Geometry check sheet. Reference: the model listing, model coordinates, mm. Face numbers are marked on the shaded views. A direction names the side the tool comes from. Round coordinates to 2 decimals unless told otherwise and drop trailing zeros. Write each loop counter-clockwise with the first axis right and the second up, starting at its lowest first coordinate (ties: lowest second). Pieces come first, ordered by that corner, then holes. Notation, with made-up numbers: M 3.5,-12.5 L 57.5,-12.5 A29 ccw 57.5,11.5 Z; hole C 40.25,-9.75 d5. An arc over 180 degrees is marked long. Put each result on its own line as item: value. Start each with the question number.
(1) Tool access check on the marked faces 1 and 2. Record the directions out of +Z, -Z, +X, -X, +Y, -Y that give a thin tool (end or side, any length) a straight path to the whole face; none if there is none.
(2) Material ranges on probe 1 along Y at (x, z) = (-11, -5); probe 2 along Y at (x, z) = (-11, -2.4); probe 3 along X at (y, z) = (10, -6.5), recorded low to high.
(3) Gauge pin test, flat ends, axial feed: pin 1 (12 mm diameter, centred on y = 13.5, z = -27, fed in from -X); pin 2 (1.5 mm diameter, centred on x = -31.5, y = 13, fed in from +Z); pin 3 (6.5 mm diameter, centred on y = 13, z = -5.5, fed in from -X). Record the tip position at first contact, or that the pin passes through.
(4) Section check A-A on y = 10. Record the cut outline in (x, z).
(5) Section check B-B on x = -11. Record the cut outline in (y, z).
(6) Section check C-C on y = 3.5. Record the cut outline in (x, z).
(7) Section check D-D on z = -9. Record the cut outline in (x, y), then the cut area to 3 significant figures.
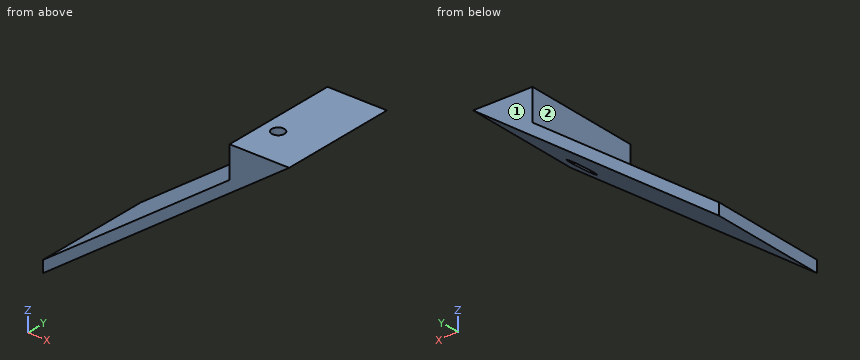
from build123d import *

# Parameters (mm, degrees)
EXTRUDE_1_DEPTH     = 30
SKETCH_2_R          = 1.6
CUT_EXTRUDE_1_DEPTH = 83.29890272
CUT_EXTRUDE_2_REACH = 82.696
SKETCH_3_R          = 3


with BuildPart() as part:
    # 草图1 → 凸台-拉伸1 (new body)
    with BuildSketch(Plane(origin=(0, 0, 0), x_dir=(1, 0, 0), z_dir=(0, 1, 0))):
        Polygon((0, 0), (-62, 45.045636736), (-62, 42.07907359), (-15, 7.931574774), (-15, 0), align=None)
    extrude(amount=EXTRUDE_1_DEPTH)

    # 草图2 → 切除-拉伸1 (cut, through all)
    with BuildSketch(Plane.XY):
        with Locations((-11, 10)):
            Circle(SKETCH_2_R)
    extrude(amount=-CUT_EXTRUDE_1_DEPTH, mode=Mode.SUBTRACT)

    # 切除-拉伸2: up to this plane
    cut_extrude_2_end = Plane(origin=(0, 30, 0), z_dir=(-0.5877852522924716, 0, 0.8090169943749486))
    # 草图3 → 切除-拉伸2 (cut, up to the surface)
    with BuildSketch(Plane.XY.offset(-3), mode=Mode.PRIVATE) as cut_extrude_2_sk1:
        with Locations((-11, 10)):
            Circle(SKETCH_3_R)
    cut_extrude_2_tool1 = split(extrude(cut_extrude_2_sk1.sketch, amount=-CUT_EXTRUDE_2_REACH, mode=Mode.PRIVATE), bisect_by=cut_extrude_2_end, keep=Keep.BOTH, mode=Mode.PRIVATE)
    add(cut_extrude_2_tool1.solids().sort_by_distance((-11, 10, -3))[0], mode=Mode.SUBTRACT)


solid = part.part
Answers follow:
1. face 1: +Z, -Z, +X, -X, +Y
1. face 2: +Z, -X, +Y, -Y
2. probe 1: y = 0 to 7, 13 to 30
2. probe 2: y = 0 to 8.4, 11.6 to 30
2. probe 3: x = -15 to -14
3. pin 1: stops at x = -49.5
3. pin 2: stops at z = -19.37
3. pin 3: stops at x = -16.13
4. outline: M -62,-45.05 L -14,-10.17 L -14,-3 L -12.6,-3 L -12.6,0 L -15,0 L -15,-7.93 L -62,-42.08 Z; M -9.4,-3 L -8,-3 L -8,-5.81 L 0,0 L -9.4,0 Z
5. outline: M 0,-7.99 L 7,-7.99 L 7,-3 L 8.4,-3 L 8.4,0 L 0,0 Z; M 11.6,-3 L 13,-3 L 13,-7.99 L 30,-7.99 L 30,0 L 11.6,0 Z
6. outline: M -62,-45.05 L 0,0 L -15,0 L -15,-7.93 L -62,-42.08 Z
7. outline: M -16.47,0 L -12.39,0 L -12.39,7.34 A3 cw -12.39,12.66 L -12.39,30 L -16.47,30 Z
7. area: 116 mm^2
